Work out the finished part from the listing and answer in its coordinate system (mm). A direction names the side the tool comes from. Give positions to 0.01 mm unless a question says otherwise; leave off trailing zeros. Write each loop counter-clockwise with the first axis right and the second up, starting at its lowest first coordinate (ties: lowest second). Pieces come first, ordered by that corner, then holes.
1) Find section C-C (y = -8.5). Determine the outline of the cut face in (x, z).
2) Find section B-B (x = -7.75). Determine the outline of the cut face in (y, z), plus the area to 3 significant figures.
3) Find section A-A (z = -7.5). Determine the outline of the cut face in (x, y), plus the area to 3 significant figures.
4) A tool of negligible diameter and unlimited length cuts with its end or side. For faces 3 (the face through (0, 0, 0)), 4 (the face through (4.25, -9, 14)), 5 (the face through (-8.208, -1, -3)), 6 (the face through (0, -6, 12.75)), 7 (the face through (11, -10, 0)), from which of +Z, -Z, +X, -X, +Y, -Y can it reach the whole face along a straight path? Write none if from no direction.
5) Determine the mould class of faces 1 (the face through (6.554, -1, 5)), 2 (the face through (-4.25, -9, 14)) for opening direction Z: pulls with the +Z half, pulls with the -Z half, needs draft (parallel to the pull), parting line crosses it, or undercut.
6) Given pin 1 Ø10.5 at (x, z) = (-3, -6) entering from -Y; pin 2 Ø1.9 at (x, z) = (-1, -13.5) entering from -Y, each flat-ended and moving along its own axis, determine where each tip first touches the part or whether it passes through.
7) Find section D-D (x = 7.25). Determine the outline of the cut face in (y, z).
8) Straight lines are drawn through the part: probe 1 along Z at (x, y) = (-7, -4); probe 2 along X at (y, z) = (-7.5, -8.25); probe 3 along X at (y, z) = (-0.4, 10). For each, find the intervals that lie inside material, in ascending order.
```python
from build123d import *

# Parameters (mm, degrees)
SKETCH2_W           = 24.5
SKETCH2_H           = 29
BOSS_EXTRUDE1_DEPTH = 10
SKETCH3_W           = 21
SKETCH3_H           = 25.5
CUT_EXTRUDE1_DEPTH  = 8.5
SKETCH4_R           = 1.1
SKETCH4_R_2         = 1.625
SKETCH4_W           = 2.9
SKETCH4_H           = 5.4
SKETCH4_H_2         = 8.2
CUT_EXTRUDE2_DEPTH  = 22.454894546
SKETCH5_W           = 8.5
SKETCH5_H           = 2.25
CUT_EXTRUDE3_DEPTH  = 34.031235218
FILLET1_R           = 0.5
SKETCH6_W           = 1.5
SKETCH6_H           = 2
BOSS_EXTRUDE2_DEPTH = 2.7
FILLET2_R           = 0.5


with BuildPart() as part:
    # Sketch2 → Boss-Extrude1 (new body)
    with BuildSketch(Plane(origin=(0, 0, 0), x_dir=(1, 0, 0), z_dir=(0, 1, 0))):
        Rectangle(SKETCH2_W, SKETCH2_H)
    extrude(amount=-BOSS_EXTRUDE1_DEPTH)

    # Sketch3 → Cut-Extrude1 (cut)
    with BuildSketch(Plane.XZ.offset(10)):
        Rectangle(SKETCH3_W, SKETCH3_H)
    extrude(amount=-CUT_EXTRUDE1_DEPTH, mode=Mode.SUBTRACT)

    # Sketch4 → Cut-Extrude2 (cut, through all)
    with BuildSketch(Plane(origin=(0, 0, 0), x_dir=(1, 0, 0), z_dir=(0, 1, 0))):
        with Locations(Location((-7.75, -10, 0), (0, 0, 270))):
            Circle(SKETCH4_R)
        with Locations(Location((-7.75, 10, 0), (0, 0, 270))):
            Circle(SKETCH4_R)
        with Locations(Location((-1.7156, -11.0712, 0), (0, 0, 270))):
            Circle(SKETCH4_R_2)
        with Locations((-6.7576, 3.3688)):
            Rectangle(SKETCH4_W, SKETCH4_H)
        with Locations((5.1042, 4.84677)):
            Rectangle(SKETCH4_W, SKETCH4_H_2)
        with Locations((5.1042, -5.31323)):
            Rectangle(SKETCH4_W, SKETCH4_H_2)
    extrude(amount=-CUT_EXTRUDE2_DEPTH, mode=Mode.SUBTRACT)

    # Sketch5 → Cut-Extrude3 (cut, through all)
    with BuildSketch(Plane.XY.offset(14.5)):
        with Locations((0, -8.875)):
            Rectangle(SKETCH5_W, SKETCH5_H)
    extrude(amount=-CUT_EXTRUDE3_DEPTH, mode=Mode.SUBTRACT)

    # Fillet1
    fillet1_edges = [part.edges().sort_by_distance(p)[0] for p in [
        (0, 0, -14.5),
        (12.25, 0, 0),
        (0, 0, 14.5),
        (-12.25, 0, 0),
        (-12.25, -5, -14.5),
        (12.25, -5, -14.5),
        (12.25, -5, 14.5),
        (-12.25, -5, 14.5),
    ]]
    fillet(fillet1_edges, radius=FILLET1_R)

    # Sketch6 → Boss-Extrude2 (add)
    with BuildSketch(Plane.XZ.offset(1.5)):
        with Locations((-9.75, -3)):
            Rectangle(SKETCH6_W, SKETCH6_H)
        with Locations((9.75, 6.5)):
            Rectangle(SKETCH6_W, SKETCH6_H)
        with Locations((9.75, -5.5)):
            Rectangle(SKETCH6_W, SKETCH6_H)
    extrude(amount=BOSS_EXTRUDE2_DEPTH)

    # Fillet2
    fillet2_edges = [part.edges().sort_by_distance(p)[0] for p in [
        (-9.75, -1.5, -2),
        (9.75, -1.5, -6.5),
        (9.75, -1.5, 5.5),
        (-9, -1.5, -3),
        (9, -1.5, -5.5),
        (9, -1.5, 6.5),
        (-9.75, -1.5, -4),
        (-10.5, -2.85, -4),
        (-9, -2.85, -4),
        (-9, -2.85, -2),
        (-10.5, -2.85, -2),
        (9.75, -1.5, -4.5),
        (10.5, -2.85, -4.5),
        (9, -2.85, -4.5),
        (9, -2.85, -6.5),
        (10.5, -2.85, -6.5),
        (9.75, -1.5, 7.5),
        (10.5, -2.85, 7.5),
        (9, -2.85, 7.5),
        (9, -2.85, 5.5),
        (10.5, -2.85, 5.5),
    ]]
    fillet(fillet2_edges, radius=FILLET2_R)


solid = part.part
```
Results:
1. outline: (-12.25, -14) arc R0.5 ccw to (-11.75, -14.5) - (-4.25, -14.5) - (-4.25, -12.75) - (-10.5, -12.75) - (-10.5, 12.75) - (-4.25, 12.75) - (-4.25, 14.5) - (-11.75, 14.5) arc R0.5 ccw to (-12.25, 14) - close; (4.25, -14.5) - (11.75, -14.5) arc R0.5 ccw to (12.25, -14) - (12.25, 14) arc R0.5 ccw to (11.75, 14.5) - (4.25, 14.5) - (4.25, 12.75) - (10.5, 12.75) - (10.5, -12.75) - (4.25, -12.75) - close
2. outline: (-10, -14.5) - (-0.5, -14.5) arc R0.5 ccw to (0, -14) - (0, -11.1) - (-1.5, -11.1) - (-1.5, -12.75) - (-10, -12.75) - close; (-10, 12.75) - (-1.5, 12.75) - (-1.5, 11.1) - (0, 11.1) - (0, 14) arc R0.5 ccw to (-0.5, 14.5) - (-10, 14.5) - close; (-1.5, -8.9) - (0, -8.9) - (0, -6.07) - (-1.5, -6.07) - close; (-1.5, -0.67) - (0, -0.67) - (0, 8.9) - (-1.5, 8.9) - close
2. area: 58.4 mm2
3. outline: (-12.25, -10) - (-10.5, -10) - (-10.5, -1.5) - (3.65, -1.5) - (3.65, 0) - (-11.75, 0) arc R0.5 ccw to (-12.25, -0.5) - close; (6.55, -1.5) - (10.5, -1.5) - (10.5, -10) - (12.25, -10) - (12.25, -0.5) arc R0.5 ccw to (11.75, 0) - (6.55, 0) - close
3. area: 62.0 mm2
4. face 3: +Z, -Z, +X, -X, +Y
4. face 4: +Z, -Z, -Y
4. face 5: +Y, -Y
4. face 6: -Y
4. face 7: +Z, -Z, +X, -X, -Y
5. face 1: undercut
5. face 2: needs draft
6. pin 1: stops at y = -1.5
6. pin 2: stops at y = -7.75
7. outline: (-10, -14.5) - (-0.5, -14.5) arc R0.5 ccw to (0, -14) - (0, 14) arc R0.5 ccw to (-0.5, 14.5) - (-10, 14.5) - (-10, 12.75) - (-1.5, 12.75) - (-1.5, -12.75) - (-10, -12.75) - close
8. probe 1: z = -14.5 to -12.75, 12.75 to 14.5
8. probe 2: x = -12.25 to -10.5, 10.5 to 12.25
8. probe 3: x = -12.24 to -8.85, -6.65 to -2.94, -0.49 to 12.24
